Can you work these out from the model? Positions are in its coordinate system, mm. A direction names the side the tool comes from. Give positions to 0.01 mm unless a question says otherwise; leave off trailing zeros. Write each loop counter-clockwise with the first axis right and the second up, starting at its lowest first coordinate (ties: lowest second). Pieces come first, ordered by that corner, then holes. Notation, with made-up numbers: M 35.25,50 L 89.25,50 A16 ccw 89.25,54 Z; hole C 63,-8 d1. An arc over 180 degrees is marked long. Write each question's results on one line, items separated by ' | '.
from build123d import *

# Parameters (mm, degrees)
SKETCH1_R           = 60
BOSS_EXTRUDE2_DEPTH = 4
SKETCH2_R           = 20
CUT_EXTRUDE1_DEPTH  = 20.9
SKETCH3_R           = 48.468089367
BOSS_EXTRUDE3_DEPTH = 3.9
SKETCH4_R           = 59.929943569
BOSS_EXTRUDE6_DEPTH = 4
SKETCH8_R           = 20
CUT_EXTRUDE5_DEPTH  = 48
CUT_EXTRUDE6_DEPTH  = 48


with BuildPart() as part:
    # Sketch1 → Boss-Extrude2 (new body)
    with BuildSketch(Plane.XY):
        Circle(SKETCH1_R)
    extrude(amount=BOSS_EXTRUDE2_DEPTH)

    # Sketch2 → Cut-Extrude1 (cut)
    with BuildSketch(Plane.XY.offset(4)):
        Circle(SKETCH2_R)
    extrude(amount=-CUT_EXTRUDE1_DEPTH, mode=Mode.SUBTRACT)

    # Sketch3 → Boss-Extrude3 (add)
    with BuildSketch(Plane.XY.offset(4)):
        Circle(SKETCH3_R)
    extrude(amount=BOSS_EXTRUDE3_DEPTH)

    # Sketch4 → Boss-Extrude6 (add)
    with BuildSketch(Plane.XY.offset(7.9)):
        Circle(SKETCH4_R)
    extrude(amount=BOSS_EXTRUDE6_DEPTH)

    # Sketch8 → Cut-Extrude5 (cut)
    with BuildSketch(Plane.XY.offset(11.9)):
        Circle(SKETCH8_R)
    extrude(amount=-CUT_EXTRUDE5_DEPTH, mode=Mode.SUBTRACT)

    # Sketch9 → Cut-Extrude6 (cut)
    with BuildSketch(Plane.XY.offset(11.9)):
        with BuildLine():
            Line((-5.95, 19.094436362), (-5.95, 23.394436362))
            Line((-5.95, 23.394436362), (5.95, 23.394436362))
            Line((5.95, 23.394436362), (5.95, 19.094436362))
            ThreePointArc((5.95, 19.094436362), (0, 20), (-5.95, 19.094436362))
        make_face()
    extrude(amount=-CUT_EXTRUDE6_DEPTH, mode=Mode.SUBTRACT)


solid = part.part
Item 1: If I drill on line 1 (Z direction, x = 47, y = 34); line 2 (Y direction, x = 0, z = 6.75); line 3 (X direction, y = -1.5, z = 2.75), over which ranges is the centre line in solid material (lowest first)? Write a range as from..to.
Geometry says:
line 1: z = 0..4, 7.9..11.9 | line 2: y = -48.47..-20, 23.39..48.47 | line 3: x = -59.98..-19.94, 19.94..59.98
Item 2: For faces 1 (the face through (26, 1, 0)), 2 (the face through (-5.95, 21, 6)), 3 (the face through (49, 0, 4)), which set-ups out of +Z, -Z, +X, -X, +Y, -Y let a thin tool reach every point of the face, with its end or its side?
Geometry says:
face 1: -Z, +X, -X, +Y, -Y | face 2: +Z, -Z | face 3: none
Item 3: I'm going to push flat-ended pins straight in: pin 1 (10 mm diameter, centred on x = -44.5, y = 6, fed in from -Z); pin 2 (3.5 mm diameter, centred on y = 20.5, z = 8, fed in from -X); pin 3 (4 mm diameter, centred on y = -3.5, z = 9, fed in from +X); pin 4 (4.5 mm diameter, centred on y = 21, z = 5.5, fed in from +X). Where does each tip first touch, or does it pass through?
Geometry says:
pin 1: stops at z = 0 | pin 2: stops at x = -56.92 | pin 3: stops at x = 59.91 | pin 4: stops at x = 56.8
Item 4: I want a section at C-C, the plane z = 10. Please give me the cut outline in (x, y), and give its area (3 significant figures).
Geometry says:
outline: C 0,0 d119.86; hole M -5.95,19.09 A20 ccw long 5.95,19.09 L 5.95,23.39 L -5.95,23.39 Z | area: 9,980 mm2
Item 5: Thinking about a two-plate mould opening in X: for faces 4 (the face through (49, 0, 7.9)), 5 (the face through (26.056, 40.868, 5.923)), 6 (the face through (0, 23.394, 6)), which applies, +X half, -X half, draft (parallel to the pull), parting line (faces both ways), or undercut?
Geometry says:
face 4: draft | face 5: parting line | face 6: undercut
Item 6: I want a section at B-B, the plane y = 0. Please give me the cut outline in (x, z).
Geometry says:
outline: M -60,0 L -20,0 L -20,11.9 L -59.93,11.9 L -59.93,7.9 L -48.47,7.9 L -48.47,4 L -60,4 Z; M 20,0 L 60,0 L 60,4 L 48.47,4 L 48.47,7.9 L 59.93,7.9 L 59.93,11.9 L 20,11.9 Z
Item 7: I want a section at D-D, the plane y = -37. Please give me the cut outline in (x, z).
Geometry says:
outline: M -47.23,0 L 47.23,0 L 47.23,4 L 31.31,4 L 31.31,7.9 L 47.14,7.9 L 47.14,11.9 L -47.14,11.9 L -47.14,7.9 L -31.31,7.9 L -31.31,4 L -47.23,4 Z
Item 8: I want a section at A-A, the plane x = 0. Please give me the cut outline in (y, z).
Geometry says:
outline: M -60,0 L -20,0 L -20,11.9 L -59.93,11.9 L -59.93,7.9 L -48.47,7.9 L -48.47,4 L -60,4 Z; M 23.39,0 L 60,0 L 60,4 L 48.47,4 L 48.47,7.9 L 59.93,7.9 L 59.93,11.9 L 23.39,11.9 Z
